from build123d import *

# Parameters (mm, degrees)
F1_DEPTH  = 7.5
F3_DEPTH  = 4
F5_R      = 3.5
F6_DEPTH  = 3
F7_R      = 5
F8_DEPTH  = 2
F4_W      = 60
F4_H      = 35
F10_DEPTH = 2


# Not quite as in the source:
# - a fillet or chamfer that OpenCascade refuses, or shapes differently, is made with other operations: its cross-section is extruded or revolved along the edge and cut away or added


with BuildPart() as f1:
    # F0 (on Right) → F1 (new body, symmetric)
    with BuildSketch(Plane.YZ):
        with BuildLine():
            Line((-34.8711436077, -24.0259013658), (-30.9017617255, -30))
            Line((-30.9017617255, -30), (0, -30))
            Line((0, -30), (0, 0))
            Line((0, 0), (-52.5, 0))
            Line((-52.5, 0), (-52.5, -18.7762488504))
            ThreePointArc((-52.5, -18.7762488504), (-51.1634624835, -19.4917800985), (-49.6902439515, -19.8494736223))
            Line((-49.6902439515, -19.8494736223), (-46.2112579103, -20.2390480822))
            Line((-46.2112579103, -20.2390480822), (-39.9225158206, -20.9432570884))
            ThreePointArc((-39.9225158206, -20.9432570884), (-37.0550608987, -21.9245400717), (-34.8711436077, -24.0259013658))
        make_face()
        with BuildLine():
            Line((0, 0), (0, -30))
            Line((0, -30), (30.9017617255, -30))
            Line((30.9017617255, -30), (34.8711436077, -24.0259013658))
            ThreePointArc((34.8711436077, -24.0259013658), (37.0550608987, -21.9245400717), (39.9225158206, -20.9432570884))
            Line((39.9225158206, -20.9432570884), (46.2112579103, -20.2390480822))
            Line((46.2112579103, -20.2390480822), (49.6902439515, -19.8494736223))
            ThreePointArc((49.6902439515, -19.8494736223), (51.1634624835, -19.4917800985), (52.5, -18.7762488504))
            Line((52.5, -18.7762488504), (52.5, 0))
            Line((52.5, 0), (0, 0))
        make_face()
        with BuildLine():
            Line((-52.5, 0), (0, 0))
            Line((0, 0), (0, 30))
            Line((0, 30), (-30.9017617255, 30))
            Line((-30.9017617255, 30), (-34.8711436077, 24.0259013658))
            ThreePointArc((-34.8711436077, 24.0259013658), (-37.0550608987, 21.9245400717), (-39.9225158206, 20.9432570884))
            Line((-39.9225158206, 20.9432570884), (-46.2112579103, 20.2390480822))
            Line((-46.2112579103, 20.2390480822), (-49.6902439515, 19.8494736223))
            ThreePointArc((-49.6902439515, 19.8494736223), (-51.1634624835, 19.4917800985), (-52.5, 18.7762488504))
            Line((-52.5, 18.7762488504), (-52.5, 0))
        make_face()
        with BuildLine():
            Line((0, 30), (0, 0))
            Line((0, 0), (52.5, 0))
            Line((52.5, 0), (52.5, 18.7762488504))
            ThreePointArc((52.5, 18.7762488504), (51.1634624835, 19.4917800985), (49.6902439515, 19.8494736223))
            Line((49.6902439515, 19.8494736223), (46.2112579103, 20.2390480822))
            Line((46.2112579103, 20.2390480822), (39.9225158206, 20.9432570884))
            ThreePointArc((39.9225158206, 20.9432570884), (37.0550608987, 21.9245400717), (34.8711436077, 24.0259013658))
            Line((34.8711436077, 24.0259013658), (30.9017617255, 30))
            Line((30.9017617255, 30), (0, 30))
        make_face()
        with BuildLine():
            Line((58.7885477615, 0), (52.5, 0))
            Line((52.5, 0), (52.5, -18.7762488504))
            ThreePointArc((52.5, -18.7762488504), (53.448824854, -17.9374222983), (54.2004466552, -16.9181268278))
            ThreePointArc((54.2004466552, -16.9181268278), (57.6211742241, -8.7646119013), (58.7885477615, 0))
        make_face()
        with BuildLine():
            Line((52.5, 18.7762488504), (52.5, 0))
            Line((52.5, 0), (58.7885477615, 0))
            ThreePointArc((58.7885477615, 0), (57.6211742241, 8.7646119013), (54.2004466552, 16.9181268278))
            ThreePointArc((54.2004466552, 16.9181268278), (53.448824854, 17.9374222983), (52.5, 18.7762488504))
        make_face()
        with BuildLine():
            Line((-58.7885477615, 0), (-52.5, 0))
            Line((-52.5, 0), (-52.5, 18.7762488504))
            ThreePointArc((-52.5, 18.7762488504), (-53.448824854, 17.9374222983), (-54.2004466552, 16.9181268278))
            ThreePointArc((-54.2004466552, 16.9181268278), (-57.6211742241, 8.7646119013), (-58.7885477615, 0))
        make_face()
        with BuildLine():
            Line((-52.5, -18.7762488504), (-52.5, 0))
            Line((-52.5, 0), (-58.7885477615, 0))
            ThreePointArc((-58.7885477615, 0), (-57.6211742241, -8.7646119013), (-54.2004466552, -16.9181268278))
            ThreePointArc((-54.2004466552, -16.9181268278), (-53.448824854, -17.9374222983), (-52.5, -18.7762488504))
        make_face()
    extrude(amount=F1_DEPTH, both=True)

    # F2 (on Right) → F3 (join, symmetric)
    with BuildSketch(Plane.YZ):
        with BuildLine():
            Line((29.7115407884, 26.9230790436), (29.7115407884, 18.846154213))
            Line((29.7115407884, 18.846154213), (46.6346181929, 18.846154213))
            Line((46.6346181929, 18.846154213), (46.6346181929, 22.9230790436))
            ThreePointArc((46.6346181929, 22.9230790436), (45.4630453177, 25.7515061684), (42.6346181929, 26.9230790436))
            Line((42.6346181929, 26.9230790436), (29.7115407884, 26.9230790436))
        make_face()
        with BuildLine():
            Line((-29.7115407884, 18.846154213), (-29.7115407884, 26.9230790436))
            Line((-29.7115407884, 26.9230790436), (-42.6346181929, 26.9230790436))
            ThreePointArc((-42.6346181929, 26.9230790436), (-45.4630453177, 25.7515061684), (-46.6346181929, 22.9230790436))
            Line((-46.6346181929, 22.9230790436), (-46.6346181929, 18.846154213))
            Line((-46.6346181929, 18.846154213), (-29.7115407884, 18.846154213))
        make_face()
    extrude(amount=F3_DEPTH, both=True)

    # F5 (on face) → F6 (join)
    with BuildSketch(Plane(origin=(-7.5, 0, 0), x_dir=(0, -1, 0), z_dir=(-1, 0, 0))):
        with Locations((-43.3653853834, -9.6153849736)):
            Circle(F5_R)
    extrude(amount=F6_DEPTH)

    # F7 (on face) → F8 (join)
    with BuildSketch(Plane(origin=(-10.5, 0, 0), x_dir=(0, -1, 0), z_dir=(-1, 0, 0))):
        with Locations((-43.3653853834, -9.6153849736)):
            Circle(F7_R)
    extrude(amount=F8_DEPTH)

    # F9: fillet of radius 5 on 1 edges, made by hand

    # F9_s1 → F9_t2 (revolve, cut)
    with BuildSketch(Plane.XY.offset(-9.6153849736)):
        with BuildLine():
            ThreePointArc((-10.5, 38.3653853834), (-11.972135955, 40.1293174059), (-12.5, 42.3653853834))
            Line((-12.5, 42.3653853834), (-12.5, 38.3653853834))
            Line((-12.5, 38.3653853834), (-10.5, 38.3653853834))
        make_face()
    revolve(axis=Axis((-12.5, 43.3653853834, -9.6153849736), (-1, 0, 0)), mode=Mode.SUBTRACT)

    # F4 (on face) → F10 (cut)
    with BuildSketch(Plane(origin=(-7.5, 0, 0), x_dir=(0, -1, 0), z_dir=(-1, 0, 0))):
        Rectangle(F4_W, F4_H)
    extrude(amount=-F10_DEPTH, mode=Mode.SUBTRACT)


solid = f1.part
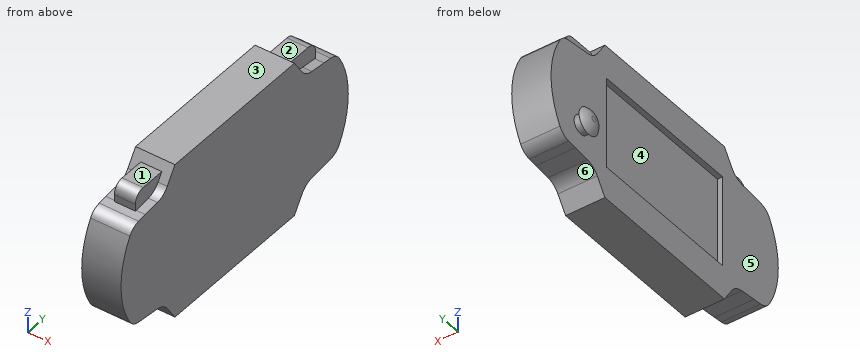
Source: CAD feature listing. Evaluate the final solid. Frame: model axes, mm. Face numbers are marked on the shaded views. A direction names the side the tool comes from. Give positions to 0.01 mm unless a question says otherwise; leave off trailing zeros. Write each loop counter-clockwise with the first axis right and the second up, starting at its lowest first coordinate (ties: lowest second). Pieces come first, ordered by that corner, then holes. Notation, with made-up numbers: (-18, -25.75) -> (8, -25.75) arc R29 ccw to (8, 9.25) -> close; hole circle Ø4 at (70.25, -21). An arc over 180 degrees is marked (long way). Return JSON: item names as keys, results as strings. Group by question number.
1. Section A-A, the plane y = -27.5. Output: boundary loops of the cut face in (x, z), then the cut area to 3 significant figures.
2. Pin query (flat end, axial travel): pin 1 Ø2 at (x, z) = (-2, 22) entering from -Y; pin 2 Ø3 at (y, z) = (-45.5, 9.5) entering from -X; pin 3 Ø9 at (x, y) = (-0.5, -36) entering from +Z. Return the tip coordinate at first contact, or that it passes through.
3. Mould query, pull axis Y, two halves, no side actions, for the marked faces 4, 5 and 6. Classes: +Y half, -Y half, draft (parallel to the pull), parting line (faces both ways), or undercut.
4. Access query for the marked faces 1, 2 and 3. Directions: +Z, -Z, +X, -X, +Y, -Y. A direction counts if a zero-diameter tool reaches every point of the face in a straight line with its end or side. Return the directions, or none.
5. Section C-C, the plane z = 14. Output: boundary loops of the cut face in (x, y).
6. Section B-B, the plane x = 5.25. Output: boundary loops of the cut face in (y, z).
7. Material intervals for line 1 (X direction, y = 28, z = 2); line 2 (X direction, y = -50.5, z = 17); line 3 (Y direction, x = -6, z = 6.5), sorted ascending. Write a range as from..to.
Determined:
{
 "1": {"outline": "(-7.5, -30) -> (7.5, -30) -> (7.5, 30) -> (-7.5, 30) -> (-7.5, 17.5) -> (-5.5, 17.5) -> (-5.5, -17.5) -> (-7.5, -17.5) -> close", "area": "830 mm2"},
 "2": {"pin 1": "stops at y = -46.63", "pin 2": "stops at x = -7.5", "pin 3": "stops at z = 29.1"},
 "3": {"face 4": "undercut", "face 5": "draft", "face 6": "+Y half"},
 "4": {"face 1": "+Z, +X, -X, -Y", "face 2": "+Z, +X, -X, +Y", "face 3": "+Z, +X, -X, +Y, -Y"},
 "5": {"outline": "(-7.5, -55.72) -> (7.5, -55.72) -> (7.5, 55.72) -> (-7.5, 55.72) -> (-7.5, 30) -> (-5.5, 30) -> (-5.5, -30) -> (-7.5, -30) -> close"},
 "6": {"outline": "(-54.2, -16.92) arc R6 ccw to (-49.69, -19.85) -> (-39.92, -20.94) arc R7 cw to (-34.87, -24.03) -> (-30.9, -30) -> (30.9, -30) -> (34.87, -24.03) arc R7 cw to (39.92, -20.94) -> (49.69, -19.85) arc R6 ccw to (54.2, -16.92) arc R33.49 ccw to (54.2, 16.92) arc R6 ccw to (49.69, 19.85) -> (39.92, 20.94) arc R7 cw to (34.87, 24.03) -> (30.9, 30) -> (-30.9, 30) -> (-34.87, 24.03) arc R7 cw to (-39.92, 20.94) -> (-49.69, 19.85) arc R6 ccw to (-54.2, 16.92) arc R33.49 ccw to start"},
 "7": {"line 1": "x = -5.5..7.5", "line 2": "x = -7.5..7.5", "line 3": "y = -58.15..-30, 30..58.15"}
}
